Could you check a few things on this model? Use its own coordinates, in mm. Coordinates: 2 decimals unless noted, no trailing zeros. Write each loop counter-clockwise with the first axis right and the second up, starting at its lowest first coordinate (ties: lowest second). Pieces come first, ordered by that corner, then holes.
Item 1: I want a section at A-A on z = 40. Please give me the cut outline in (x, y), then the cut area to 3 significant figures.
Item 2: I want a section at C-C on x = 67. Please give me the cut outline in (y, z).
Item 3: If I drill on probe 1 along X at (y, z) = (1.1, -54); probe 2 along X at (y, z) = (1.85, 45); probe 3 along Z at (x, y) = (-36, 2.95), over which ranges is the centre line in solid material (lowest first)?
Item 4: For P1, Ø1.5, axis at y = 2, z = 43, coming from the +X side; P2, Ø2.5, axis at x = 27.47, z = -50.39, coming from the +Y side; P3, Ø0.9, axis at y = 2, z = 24, coming from the +X side, each with a flat end and sliding along its axis, tell me the tip position at first contact or that it passes through.
Item 5: I want a section at B-B on y = 1.95. State how many separate pieces and enclosed holes the cut face has, then the cut area to 3 significant figures.
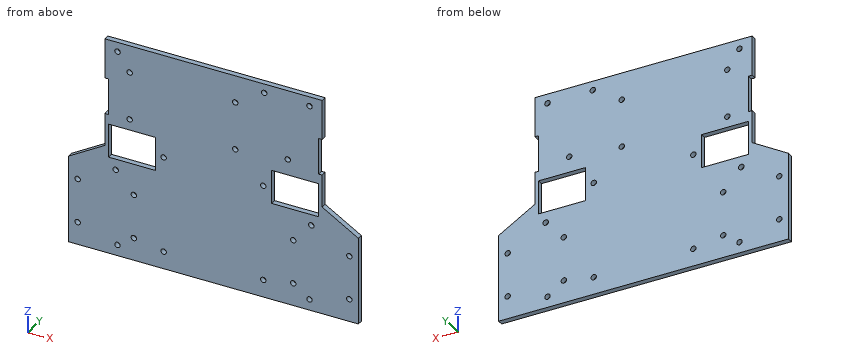
from build123d import *

# Parameters (mm, degrees)
SKETCH1_W           = 120
SKETCH1_H           = 120
BOSS_EXTRUDE1_DEPTH = 3
SKETCH2_R           = 1.5
CUT_EXTRUDE1_DEPTH  = 101.04498988
SKETCH3_R           = 1.5
CUT_EXTRUDE3_DEPTH  = 101.04498988
SKETCH4_R           = 1.5
CUT_EXTRUDE4_DEPTH  = 101.04498988
SKETCH6_R           = 1.525
CUT_EXTRUDE7_DEPTH  = 101.04498988
SKETCH10_W          = 25.970420931
SKETCH10_H          = 18.602515671
CUT_EXTRUDE9_DEPTH  = 5
SKETCH11_R          = 1.5
CUT_EXTRUDE10_DEPTH = 5
SKETCH12_W          = 2.05
SKETCH12_H          = 20
CUT_EXTRUDE11_DEPTH = 10


with BuildPart() as part:
    # Sketch1 → Boss-Extrude1 (new body)
    with BuildSketch(Plane(origin=(0, 0, 0), x_dir=(1, 0, 0), z_dir=(0, 1, 0))):
        Rectangle(SKETCH1_W, SKETCH1_H)
        Polygon((-80, 11.791828604), (-60, 0), (-60, 60), (-80, 60), align=None)
        Polygon((80, 60), (60, 60), (60, 0), (80, 11.791828604), align=None)
    extrude(amount=BOSS_EXTRUDE1_DEPTH)

    # Sketch2 → Cut-Extrude1 (cut, through all)
    with BuildSketch(Plane(origin=(0, 3, 0), x_dir=(1, 0, 0), z_dir=(0, 1, 0))):
        with Locations(Location((28, -55, 0), (0, 0, 270))):
            Circle(SKETCH2_R)
        with Locations(Location((41, -21.300528194, 0), (0, 0, 270))):
            Circle(SKETCH2_R)
        with Locations(Location((-46.29, -45, 0), (0, 0, 270))):
            Circle(SKETCH2_R)
        with Locations(Location((12, -45, 0), (0, 0, 270))):
            Circle(SKETCH2_R)
        with Locations(Location((-46.29, -18.6, 0), (0, 0, 270))):
            Circle(SKETCH2_R)
        with Locations(Location((12, -18.6, 0), (0, 0, 270))):
            Circle(SKETCH2_R)
    extrude(amount=-CUT_EXTRUDE1_DEPTH, mode=Mode.SUBTRACT)

    # Sketch3 → Cut-Extrude3 (cut, through all)
    with BuildSketch(Plane(origin=(0, 3, 0), x_dir=(1, 0, 0), z_dir=(0, 1, 0))):
        with Locations(Location((-27.529579069, 50.385555627, 0), (0, 0, 270))):
            Circle(SKETCH3_R)
        with Locations(Location((-27.529579069, -2.614444373, 0), (0, 0, 90))):
            Circle(SKETCH3_R)
        with Locations(Location((27.470420931, -2.614444373, 0), (0, 0, 270))):
            Circle(SKETCH3_R)
        with Locations(Location((27.470420931, 50.385555627, 0), (0, 0, 90))):
            Circle(SKETCH3_R)
    extrude(amount=-CUT_EXTRUDE3_DEPTH, mode=Mode.SUBTRACT)

    # Sketch4 → Cut-Extrude4 (cut, through all)
    with BuildSketch(Plane(origin=(0, 3, 0), x_dir=(1, 0, 0), z_dir=(0, 1, 0))):
        with Locations(Location((-75, 23.24, 0), (0, 0, 270))):
            Circle(SKETCH4_R)
        with Locations(Location((-75, 47.5, 0), (0, 0, 270))):
            Circle(SKETCH4_R)
        with Locations(Location((-44, 23.24, 0), (0, 0, 90))):
            Circle(SKETCH4_R)
        with Locations(Location((-44, 47.5, 0), (0, 0, 90))):
            Circle(SKETCH4_R)
        with Locations(Location((44, 47.5, 0), (0, 0, 270))):
            Circle(SKETCH4_R)
        with Locations(Location((44, 23.24, 0), (0, 0, 270))):
            Circle(SKETCH4_R)
        with Locations(Location((75, 23.24, 0), (0, 0, 90))):
            Circle(SKETCH4_R)
        with Locations(Location((75, 47.5, 0), (0, 0, 90))):
            Circle(SKETCH4_R)
    extrude(amount=-CUT_EXTRUDE4_DEPTH, mode=Mode.SUBTRACT)

    # Sketch6 → Cut-Extrude7 (cut, through all)
    with BuildSketch(Plane(origin=(0, 3, 0), x_dir=(1, 0, 0), z_dir=(0, 1, 0))):
        with Locations(Location((-53, -54.8, 0), (0, 0, 270))):
            Circle(SKETCH6_R)
        with Locations(Location((53, -54.8, 0), (0, 0, 90))):
            Circle(SKETCH6_R)
        with Locations(Location((-54, 12.002515671, 0), (0, 0, 270))):
            Circle(SKETCH6_R)
        with Locations(Location((54, 12.002515671, 0), (0, 0, 90))):
            Circle(SKETCH6_R)
    extrude(amount=-CUT_EXTRUDE7_DEPTH, mode=Mode.SUBTRACT)

    # Sketch10 → Cut-Extrude9 (cut)
    with BuildSketch(Plane(origin=(0, 3, 0), x_dir=(1, 0, 0), z_dir=(0, 1, 0))):
        with Locations((-45.014789535, -3.298742165)):
            Rectangle(SKETCH10_W, SKETCH10_H)
        with Locations((45.014789535, -3.298742165)):
            Rectangle(SKETCH10_W, SKETCH10_H)
    extrude(amount=-CUT_EXTRUDE9_DEPTH, mode=Mode.SUBTRACT)

    # Sketch11 → Cut-Extrude10 (cut)
    with BuildSketch(Plane(origin=(0, 3, 0), x_dir=(1, 0, 0), z_dir=(0, 1, 0))):
        with Locations(Location((-53, 54, 0), (0, 0, 270))):
            Circle(SKETCH11_R)
        with Locations(Location((53, 54, 0), (0, 0, 270))):
            Circle(SKETCH11_R)
    extrude(amount=-CUT_EXTRUDE10_DEPTH, mode=Mode.SUBTRACT)

    # Sketch12 → Cut-Extrude11 (cut)
    with BuildSketch(Plane(origin=(0, 3, 0), x_dir=(1, 0, 0), z_dir=(0, 1, 0))):
        with Locations((-58.975, -28)):
            Rectangle(SKETCH12_W, SKETCH12_H)
        with Locations((58.975, -28)):
            Rectangle(SKETCH12_W, SKETCH12_H)
    extrude(amount=-CUT_EXTRUDE11_DEPTH, mode=Mode.SUBTRACT)


solid = part.part
Response values:
1. outline: (-60, 0) - (60, 0) - (60, 3) - (-60, 3) - close
1. area: 360 mm2
2. outline: (0, -60) - (3, -60) - (3, -4.13) - (0, -4.13) - close
3. probe 1: x = -80 to -54.5, -51.5 to 51.5, 54.5 to 80
3. probe 2: x = -60 to -47.79, -44.79 to 10.5, 13.5 to 60
3. probe 3: z = -60 to -6, 12.6 to 60
4. P1: stops at x = 60
4. P2: passes through
4. P3: stops at x = 57.95
5. separate pieces: 1
5. enclosed holes: 26
5. area: 15,300 mm2
